```python
from build123d import *

# Parameters (mm, degrees)
F2_R            = 23.3007414911
F3_DEPTH        = 16
F5_DEPTH        = 16
F5_COPIES_COUNT = 30
F7_R            = 23.3007414911
F8_DEPTH        = 1.5


# Not quite as in the source:
# - a feature of the source that left no trace in its solid (it failed there, or was rolled back) is left out
# - a pattern or mirror of a feature is missing from the dataset's text; its kind, count and spacing are read off the source's solid


with BuildPart() as f3:
    # F2 (on Top) → F3 (new body)
    with BuildSketch(Plane.XY):
        Circle(F2_R)
    extrude(amount=F3_DEPTH)

    # F4 (on face) → F5 (cut, through all)
    with BuildSketch(Plane.XY.offset(16)):
        with BuildLine():
            ThreePointArc((-1.9882155288, 23.2157608758), (-1.6432389463, 23.0968097974), (-1.4998597988, 22.7612496365))
            ThreePointArc((-1.4998597988, 22.7612496365), (0, 21.2407414911), (1.4998597988, 22.7612496365))
            ThreePointArc((1.4998597988, 22.7612496365), (1.6432389463, 23.0968097974), (1.9882155288, 23.2157608758))
            ThreePointArc((1.9882155288, 23.2157608758), (0, 23.3007414911), (-1.9882155288, 23.2157608758))
        make_face()
    f5 = extrude(amount=-F5_DEPTH, mode=Mode.SUBTRACT)

    # F5_copies: F5 ×30 about axis
    f5_copies_axis = Axis((0, 0, 0), (0, 0, 1))
    for i in range(1, F5_COPIES_COUNT):
        add(f5.rotate(f5_copies_axis, i * 360 / F5_COPIES_COUNT), mode=Mode.SUBTRACT)

    # F7 (on face) → F8 (join)
    with BuildSketch(Plane.XY.offset(16)):
        Circle(F7_R)
    extrude(amount=F8_DEPTH)


solid = f3.part
```
Here's how the part is built. I have some questions about the finished solid (model axes, mm). A direction names the side the tool comes from. Round coordinates to 2 decimals unless told otherwise and drop trailing zeros. Loops run counter-clockwise (first coordinate to the right, second up) from the corner with the lowest first, then second, coordinate; pieces in that order, holes last. Notation, with made-up numbers: (-14.5, 45.5) -> (-10.5, 45.5) arc R15 ccw to (-10.5, 60.5) -> close; hole circle Ø2 at (87.5, 70.25). An arc over 180 degrees is marked (long way). Answer as CSV lines item,"result".
1. Thinking about a two-plate mould opening in X: for faces 1 (the face through (-20.19, -6.6, 8.11)), 2 (the face through (0, 0, 17.5)), which applies, released by +X, released by -X, zero draft, split by the parting line, or undercut?
Final values:
face 1,"undercut"
face 2,"zero draft"
2. If we section it at A-A on x = 0: Please give me the cut outline in (y, z), plus the area to 3 significant figures.
Final values:
outline,"(-23.3, 16) -> (-21.24, 16) -> (-21.24, 0) -> (21.24, 0) -> (21.24, 16) -> (23.3, 16) -> (23.3, 17.5) -> (-23.3, 17.5) -> close"
area,"750 mm^2"
3. If we section it at B-B on y = 15: Please give me the cut outline in (x, z).
Final values:
outline,"(-17.83, 16) -> (-15.42, 16) -> (-15.42, 0) -> (15.42, 0) -> (15.42, 16) -> (17.83, 16) -> (17.83, 17.5) -> (-17.83, 17.5) -> close"
4. Which directions (+Z, -Z, +X, -X, +Y, -Y) give clear straight access to the entire face, cutting with the end or side of a thin tool? Please do faces 3 (the face through (-8.61, -19.42, 8.11)), 4 (the face through (0, -22, 16)).
Final values:
face 3,"-Z"
face 4,"-Z, -Y"
5. For pin 1 (8 mm diameter, centred on y = -16.5, z = 9, fed in from -X); pin 2 (1 mm diameter, centred on x = 6.5, z = 3, fed in from +Y); pin 3 (3 mm diameter, centred on x = 13.5, z = 9.5, fed in from +Y); pin 4 (2.5 mm diameter, centred on x = -16.5, y = 16, fed in from -Z), each with a flat end and sliding along its axis, tell me the tip position at first contact or that it passes through.
Final values:
pin 1,"stops at x = -19.19"
pin 2,"stops at y = 22.31"
pin 3,"stops at y = 19.97"
pin 4,"stops at z = 0"
6. If I drill on L1, parallel to Y at x = -18.5, z = 14.25; L2, parallel to X at y = 10, z = 6; L3, parallel to X at y = -9, z = 1.75, over which ranges is the centre line in solid material (lowest first)?
Final values:
L1,"y = -14.14 to -12.28, -10.46 to 10.46, 12.28 to 14.14"
L2,"x = -21.02 to -20.3, -19.08 to 19.08, 20.3 to 21.02"
L3,"x = -21.49 to 21.49"
